Source: CAD feature listing. Evaluate the final solid. Frame: model axes, mm. Give positions to 0.01 mm unless a question says otherwise; leave off trailing zeros. Write each loop counter-clockwise with the first axis right and the second up, starting at its lowest first coordinate (ties: lowest second). Pieces come first, ordered by that corner, then holes. Notation, with made-up numbers: (75, 8) -> (132, 8) arc R15 ccw to (132, 31) -> close; hole circle Ø10 at (-19.75, -17.75). An arc over 180 degrees is marked (long way). Write item = value, one per line.
from build123d import *

# Parameters (mm, degrees)
F1_DEPTH = 1.2
F3_DEPTH = 10
F5_DEPTH = 135
F6_R     = 5
F7_R     = 63.736196
F8_DEPTH = 1.2


with BuildPart() as f1:
    # F0 (on Top) → F1 (new body)
    with BuildSketch(Plane.XY):
        with BuildLine():
            ThreePointArc((-31.622777, -15), (0, 35), (31.622777, -15))
            Line((31.622777, -15), (41.622777, -15))
            ThreePointArc((41.622777, -15), (0, 45), (-41.622777, -15))
            Line((-41.622777, -15), (-31.622777, -15))
        make_face()
    extrude(amount=F1_DEPTH)

    # F2 (on face) → F3 (join)
    with BuildSketch(Plane.XY.offset(1.2)):
        with BuildLine():
            ThreePointArc((-31.622777, -15), (0, 35), (31.622777, -15))
            Line((31.622777, -15), (32.822777, -15))
            ThreePointArc((32.822777, -15), (0, 36.2), (-32.822777, -15))
            Line((-32.822777, -15), (-31.622777, -15))
        make_face()
    extrude(amount=F3_DEPTH)

    # F4 (on face) → F5 (join)
    with BuildSketch(Plane.XY.offset(1.2)):
        with BuildLine():
            Line((40.822777, -15), (41.622777, -15))
            ThreePointArc((41.622777, -15), (0, 45), (-41.622777, -15))
            Line((-41.622777, -15), (-40.822777, -15))
            ThreePointArc((-40.822777, -15), (0, 44.2), (40.822777, -15))
        make_face()
    extrude(amount=F5_DEPTH)

    # F6
    f6_edges = [f1.edges().sort_by_distance(p)[0] for p in [
        (-31.622777, -15, 5.6),
        (31.622777, -15, 5.6),
    ]]
    fillet(f6_edges, radius=F6_R)


with BuildPart() as f8:
    # F7 (on Top) → F8 (new body, through all)
    with BuildSketch(Plane.XY):
        Circle(F7_R)
    extrude(amount=F8_DEPTH)

    # F9: intersect F1
    add(f1.part, mode=Mode.INTERSECT)


solid = f8.part
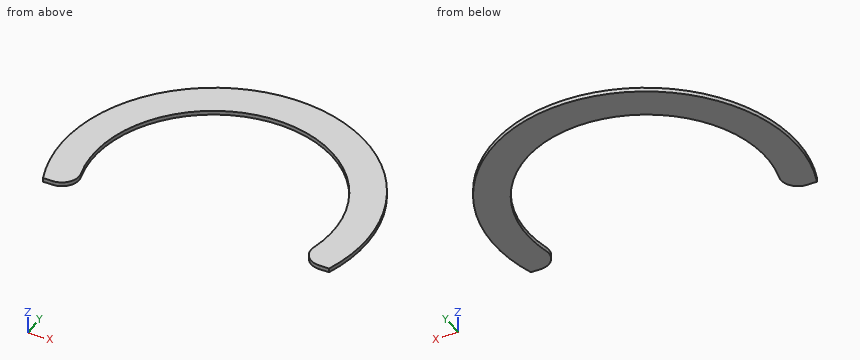
(1) Section query D-D (z = 0.6). Return loops of the section in (x, y), plus the area to 3 significant figures.
Values follow:
outline = (-41.62, -15) -> (-38.73, -15) arc R5 ccw to (-33.89, -8.75) arc R35 cw (long way) to (33.89, -8.75) arc R5 ccw to (38.73, -15) -> (41.62, -15) arc R44.44 ccw (long way) to start
area = 1,490 mm2
(2) Section query A-A (y = 11). Return loops of the section in (x, z), plus the area to 3 significant figures.
Values follow:
outline = (-43.19, 0) -> (-33.23, 0) -> (-33.23, 1.2) -> (-43.19, 1.2) -> close; (33.23, 0) -> (43.19, 0) -> (43.19, 1.2) -> (33.23, 1.2) -> close
area = 23.9 mm2
(3) Section query B-B (x = 0). Return loops of the section in (y, z).
Values follow:
outline = (35, 0) -> (45, 0) -> (45, 1.2) -> (35, 1.2) -> close
(4) Section query C-C (y = 5). Return loops of the section in (x, z).
Values follow:
outline = (-44.22, 0) -> (-34.64, 0) -> (-34.64, 1.2) -> (-44.22, 1.2) -> close; (34.64, 0) -> (44.22, 0) -> (44.22, 1.2) -> (34.64, 1.2) -> close
(5) Material intervals for line 1 (X direction, y = 0, z = 0.75); line 2 (X direction, y = -3, z = 0.6); line 3 (X direction, y = 36, z = 0.95), sorted ascending.
Values follow:
line_1 = -44.43 to -35, 35 to 44.43
line_2 = -44.29 to -34.87, 34.87 to 44.29
line_3 = -26.81 to 26.81
